```python
from build123d import *

# Parameters (mm, degrees)
F0_W      = 28.448
F0_H      = 73.406
F1_DEPTH  = 15.875
F2_W      = 28.575
F2_H      = 6.35
F3_DEPTH  = 7.874
F5_W      = 28.575
F5_H      = 6.35
F6_DEPTH  = 4.826
F8_DEPTH  = 12.7
F12_DEPTH = 40.132


with BuildPart() as f1:
    # F0 (on Front) → F1 (new body, symmetric)
    with BuildSketch(Plane.XZ):
        Rectangle(F0_W, F0_H)
    extrude(amount=F1_DEPTH, both=True)

    # F2 (on Right) → F3 (join, symmetric)
    with BuildSketch(Plane.YZ):
        Polygon((-15.875, -36.703), (-15.875, 30.353), (-44.45, 30.353), (-44.45, -32.893), (-26.924, -32.893), (-26.924, -52.4899314183), (-15.875, -41.4409314183), align=None)
        with Locations((-30.1625, 33.528)):
            Rectangle(F2_W, F2_H)
    extrude(amount=F3_DEPTH, both=True)

    # F5 (on offset) → F6 (cut)
    with BuildSketch(Plane.YZ.offset(7.874)):
        with Locations((-30.1625, 33.528)):
            Rectangle(F5_W, F5_H)
    extrude(amount=-F6_DEPTH, mode=Mode.SUBTRACT)

    # F7 (on Right) → F8 (join, symmetric)
    with BuildSketch(Plane.YZ):
        Polygon((-26.924, -32.893), (-44.45, -32.893), (-44.45, -70.0159314183), (-26.924, -52.4899314183), align=None)
    extrude(amount=F8_DEPTH, both=True)

    # F10: F1 across plane


with BuildPart() as f1_1:
    add(f1.part)
    add(f1.part.mirror(Plane.XZ))

    # F11 (on offset) → F12 (cut)
    with BuildSketch(Plane.YZ.offset(7.874)):
        with BuildLine():
            ThreePointArc((-30.226, 17.653), (-34.1773126933, 16.0163126933), (-35.814, 12.065))
            Line((-35.814, 12.065), (-35.814, -11.811))
            ThreePointArc((-35.814, -11.811), (-34.1773126933, -15.7623126933), (-30.226, -17.399))
            ThreePointArc((-30.226, -17.399), (-26.2746873067, -15.7623126933), (-24.638, -11.811))
            Line((-24.638, -11.811), (-24.638, 12.065))
            ThreePointArc((-24.638, 12.065), (-26.2746873067, 16.0163126933), (-30.226, 17.653))
        make_face()
        with BuildLine():
            ThreePointArc((30.226, -17.399), (34.1773126933, -15.7623126933), (35.814, -11.811))
            Line((35.814, -11.811), (35.814, 12.065))
            ThreePointArc((35.814, 12.065), (34.1773126933, 16.0163126933), (30.226, 17.653))
            ThreePointArc((30.226, 17.653), (26.2746873067, 16.0163126933), (24.638, 12.065))
            Line((24.638, 12.065), (24.638, -11.811))
            ThreePointArc((24.638, -11.811), (26.2746873067, -15.7623126933), (30.226, -17.399))
        make_face()
    extrude(amount=-F12_DEPTH, mode=Mode.SUBTRACT)


solid = f1_1.part
```
Input: part model. Units: mm. Frame: model coordinates. A direction names the side the tool comes from. Round coordinates to 2 decimals unless told otherwise and drop trailing zeros. Loops run counter-clockwise (first coordinate to the right, second up) from the corner with the lowest first, then second, coordinate; pieces in that order, holes last. Notation, with made-up numbers: (4, -23) - (11, -23) arc R24 ccw to (11, 11) - close; hole circle Ø5 at (26.5, 83.5). An arc over 180 degrees is marked (long way). One line per item, written item: value. Start each with the question number.
(1) Section B-B, the plane x = 5. Return loops of the section in (y, z) (3 decimals), plus the area to 3 significant figures.
(2) Draft query along Y for faces 5 (the flat face through (3.048, -30, 34)), 6 (the flat face through (0, 44.45, -28)), 7 (the flat face through (0.178, 33.538, -59.103)). Return one class per face: +Y half, -Y half, draft (parallel to the pull), parting line (faces both ways), or undercut.
(3) Ray query, line 1 (Y direction, x = -4.25, z = 11); line 2 (Y direction, x = 11, z = -46.5); line 3 (Y direction, x = -7.25, z = -13). Return the intervals inside material, ascending. Write a range as [from, to].
(4) Section A-A, the plane x = -11.5. Return loops of the section in (y, z) (3 decimals), plus the area to 3 significant figures.
(5) Section C-C, the plane z = 20.5. Return loops of the section in (x, y) (3 decimals).
(6) Section D-D, the plane y = 33.5. Return loops of the section in (x, z).
(7) Access query for faces 1 (the flat face through (0, -35.814, 0)), 2 (the flat face through (10, 26.924, -43)), 3 (the flat face through (-10, 26.924, -43)), 4 (the flat face through (5, -30, 30.353)). Directions: +Z, -Z, +X, -X, +Y, -Y. A direction counts if a zero-diameter tool reaches every point of the face in a straight line with its end or side. Return the directions, or none.
(8) Contact query for flat-ended pins moving along their axis: P1, Ø6, axis at y = -35, z = 13, coming from the -X side; P2, Ø19.5, axis at y = -34.5, z = -51.5, coming from the -X side; P3, Ø1, axis at x = -11, y = -29.5, coming from the -Z side. Output: stop coordinate, or through.
Results below:
1. outline: (-44.45, -70.016) - (-15.875, -41.441) - (-15.875, -36.703) - (15.875, -36.703) - (15.875, -41.441) - (44.45, -70.016) - (44.45, 30.353) - (15.875, 30.353) - (15.875, 36.703) - (-15.875, 36.703) - (-15.875, 30.353) - (-44.45, 30.353) - close; hole (-35.814, -11.811) arc R5.588 ccw to (-24.638, -11.811) - (-24.638, 12.065) arc R5.588 ccw to (-35.814, 12.065) - close; hole (24.638, -11.811) arc R5.588 ccw to (35.814, -11.811) - (35.814, 12.065) arc R5.588 ccw to (24.638, 12.065) - close
1. area: 6,520 mm^2
2. face 5: draft
2. face 6: +Y half
2. face 7: undercut
3. line 1: [-44.45, -35.81], [-24.64, 24.64], [35.81, 44.45]
3. line 2: [-44.45, -26.92], [26.92, 44.45]
3. line 3: [-44.45, -35.69], [-24.77, 24.77], [35.69, 44.45]
4. outline: (-44.45, -70.016) - (-26.924, -52.49) - (-26.924, -32.893) - (-44.45, -32.893) - close; (-15.875, -36.703) - (15.875, -36.703) - (15.875, 36.703) - (-15.875, 36.703) - close; (26.924, -52.49) - (44.45, -70.016) - (44.45, -32.893) - (26.924, -32.893) - close
4. area: 3,320 mm^2
5. outline: (-14.224, -15.875) - (-7.874, -15.875) - (-7.874, -44.45) - (7.874, -44.45) - (7.874, -15.875) - (14.224, -15.875) - (14.224, 15.875) - (7.874, 15.875) - (7.874, 44.45) - (-7.874, 44.45) - (-7.874, 15.875) - (-14.224, 15.875) - close
6. outline: (-12.7, -59.07) - (12.7, -59.07) - (12.7, -32.89) - (7.87, -32.89) - (7.87, -16.34) - (-7.87, -16.34) - (-7.87, -32.89) - (-12.7, -32.89) - close; (-7.87, 16.59) - (7.87, 16.59) - (7.87, 30.35) - (3.05, 30.35) - (3.05, 36.7) - (-7.87, 36.7) - close
7. face 1: +X, -X
7. face 2: +Z, -Z, +X
7. face 3: +Z, -Z, -X
7. face 4: +Z, +X, -Y
8. P1: x = -7.87
8. P2: x = -12.7
8. P3: z = -55.57
